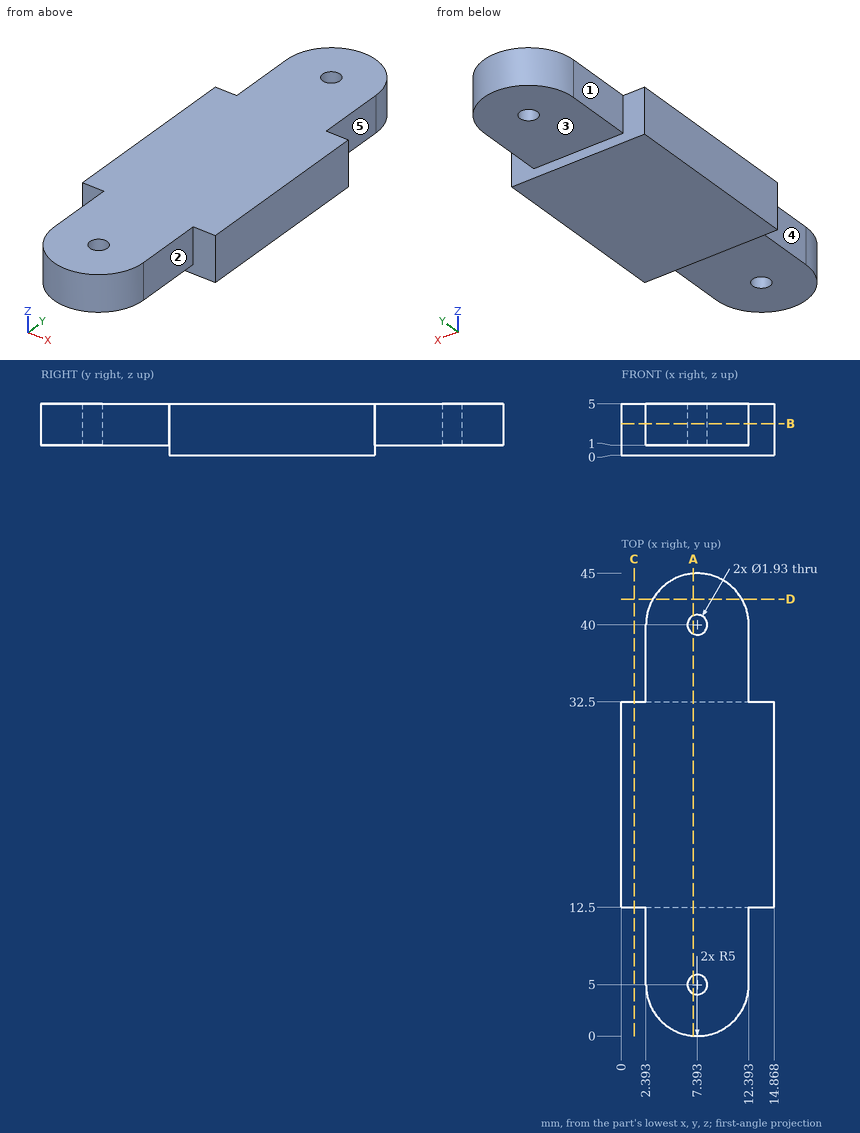
Job drawing, mm, ordinate dimensions from the low corner. One solid piece. A direction names the side the tool comes from. Give positions to 0.01 mm unless a question says otherwise; leave off trailing zeros. Loops run counter-clockwise (first coordinate to the right, second up) from the corner with the lowest first, then second, coordinate; pieces in that order, holes last.
Item 1: Flat gauge pins, fed straight in: pin 1 (3 mm diameter, centred on x = 2.5, y = 15, fed in from -Z); pin 2 (3 mm diameter, centred on x = 11, z = 1.5, fed in from -Y) (1 decimal); pin 3 (8 mm diameter, centred on x = 5, y = 5.5, fed in from -Z); pin 4 (2 mm diameter, centred on y = 35.5, z = 4, fed in from -X). Where does each tip first touch, or does it go through?
Answers follow:
pin 1: stops at z = 0
pin 2: stops at y = 0.5
pin 3: stops at z = 1
pin 4: stops at x = 2.39
Item 2: Drill centre lines: line 1 (Y direction, x = 7.5, z = 3.85); line 2 (Y direction, x = 1, z = 3.2); line 3 (X direction, y = 7, z = 4.8). Where is each one in solid material? Low to high.
Answers follow:
line 1: y = 0 to 4.04, 5.96 to 39.04, 40.96 to 45
line 2: y = 12.5 to 32.5
line 3: x = 2.39 to 12.39
Item 3: Slice it at C-C, the plane x = 1.25. List the corners of the cut face in (y, z).
Answers follow:
outline: (12.5, 0) - (32.5, 0) - (32.5, 5) - (12.5, 5) - close
Item 4: Slice it at A-A, the plane x = 7. List the corners of the cut face in (y, z) (1 decimal).
Answers follow:
outline: (0, 1) - (4.1, 1) - (4.1, 5) - (0, 5) - close; (5.9, 1) - (12.5, 1) - (12.5, 0) - (32.5, 0) - (32.5, 1) - (39.1, 1) - (39.1, 5) - (5.9, 5) - close; (40.9, 1) - (45, 1) - (45, 5) - (40.9, 5) - close
Item 5: Which spindle directions (+Z, -Z, +X, -X, +Y, -Y) get a long thin tool onto all of the face, cutting with end or side? Do the marked faces 1, 2, 3, 4 and 5. Say none if no direction does.
Answers follow:
face 1: +Z, -Z, -X, +Y
face 2: +Z, -Z, +X, -Y
face 3: -Z, +X, -X, +Y
face 4: +Z, -Z, -X, -Y
face 5: +Z, -Z, +X, +Y
Item 6: Slice it at D-D, the plane y = 42.5. List the corners of the cut face in (x, z).
Answers follow:
outline: (3.06, 1) - (11.72, 1) - (11.72, 5) - (3.06, 5) - close
Item 7: Slice it at B-B, the plane z = 3.1. List the corners of the cut face in (x, y) (1 decimal).
Answers follow:
outline: (0, 12.5) - (2.4, 12.5) - (2.4, 5) arc R5 ccw to (12.4, 5) - (12.4, 12.5) - (14.9, 12.5) - (14.9, 32.5) - (12.4, 32.5) - (12.4, 40) arc R5 ccw to (2.4, 40) - (2.4, 32.5) - (0, 32.5) - close; hole circle Ø1.9 at (7.4, 5); hole circle Ø1.9 at (7.4, 40)
